Verification items for the finished model (mm, model axes). Round coordinates to 2 decimals unless told otherwise and drop trailing zeros. Loops run counter-clockwise (first coordinate to the right, second up) from the corner with the lowest first, then second, coordinate; pieces in that order, holes last. Notation, with made-up numbers: (-16, 40) - (20, 40) arc R6 cw to (20, 51) - close; hole circle Ø9 at (16.25, -15). An arc over 180 degrees is marked (long way). Use a Markdown table: item, result. Add a question column.
Autodesk Inventor part; units mm, degrees
ref_plane "YZ Plane" through (0, 0, 0) normal (1, 0, 0) x (0, 1, 0)
ref_plane "XZ Plane" through (0, 0, 0) normal (0, 1, 0) x (-1, 0, 0)
ref_plane "XY Plane" through (0, 0, 0) normal (0, 0, 1) x (1, 0, 0)
sketch "Boceto1" plane through (0, 0, 0) normal (0, 1, 0) x (-1, 0, 0)
  line L0 (-23.8, -33.6) -> (23.8, -33.6)
  line L1 (23.8, -33.6) -> (23.8, 33.6)
  line L2 (23.8, 33.6) -> (-23.8, 33.6)
  line L3 (-23.8, 33.6) -> (-23.8, -33.6)
  line L4 (-12.4, -30.6) -> (12.9, -30.6)
  line L5 (12.4, 30.6) -> (-12.9, 30.6)
  line L6 (-23.8, 33.6) -> (-23.8, 29.4)
  circle A0 centre (-18.35, 27.65) radius 1.75
  line L7 (-16.6, 29.4) -> (-20.1, 25.9) construction
  line L8 (-20.1, 29.4) -> (-16.6, 25.9) construction
  line L9 (-12.9, 22.2) -> (-20.8, 22.2)
  line L10 (-23.8, 22.2) -> (-23.8, 33.1)
  line L11 (-12.9, 30.6) -> (-12.9, 22.2)
  line L12 (0, 33.6) -> (0, -33.6)
  line L13 (-23.8, 0) -> (23.8, 0)
  circle A1 centre (-17.85, -28.15) radius 1.75
  line L14 (-19.6, -26.4) -> (-16.1, -29.9) construction
  line L15 (-19.6, -29.9) -> (-16.1, -26.4) construction
  line L16 (-12.4, -22.7) -> (-12.4, -30.6)
  line L17 (-20.8, -22.7) -> (-12.4, -22.7)
  circle A2 centre (18.35, -27.65) radius 1.75
  line L18 (16.6, -29.4) -> (20.1, -25.9) construction
  line L19 (12.9, -22.2) -> (20.8, -22.2)
  line L20 (12.9, -30.6) -> (12.9, -22.2)
  circle A3 centre (17.85, 28.15) radius 1.75
  line L21 (19.6, 26.4) -> (16.1, 29.9) construction
  line L22 (19.6, 29.9) -> (16.1, 26.4) construction
  line L23 (12.4, 22.7) -> (12.4, 30.6)
  line L24 (20.8, 22.7) -> (12.4, 22.7)
  line L25 (20.8, -22.2) -> (20.8, 22.7)
  line L26 (-20.8, 22.2) -> (-20.8, -22.7)
  point P0 (0, 0)
  dimension "d0" = 47.6
  dimension "d1" = 67.2
  dimension "d3" = 4.2
  dimension "d5" = 3.5
  dimension "d9" = 3.5
  dimension "d11" = 3.5
extrude "Extrusión1" add sketch "Boceto1" along normal blind 2 contours L3 L13 L26 L17 L16 L4 L12 L0 | L12 L4 L20 L19 L25 L13 L1 L0 | L3 L2 L12 L5 L11 L9 L26 L13 | L13 L25 L24 L23 L5 L12 L2 L1
fillet "Empalme1" radius 8.4 4 edges at (-12.4, 1, 22.7) (12.9, 1, 22.2) (12.4, 1, -22.7) (-12.9, 1, -22.2)
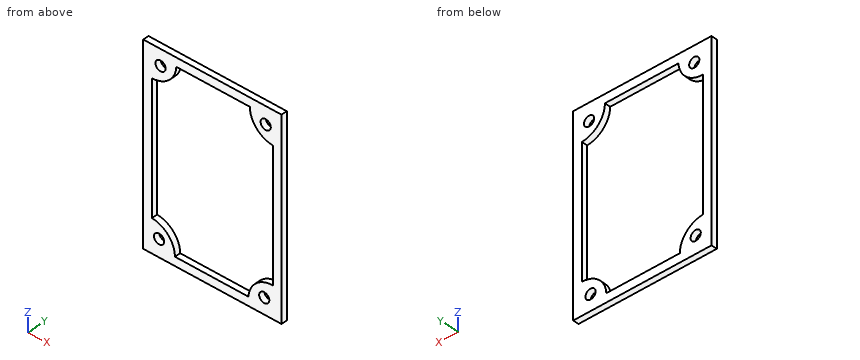
Q1. Section check D-D on x = -18.35. Record the cut outline in (y, z), plus the area to 3 significant figures.
Q2. Section check A-A on y = 0.8. State how many separate pieces and enclosed holes the cut face has, plus the area to 3 significant figures.
Q3. Section check C-C on z = -3.5. Record the cut outline in (x, y), plus the area to 3 significant figures.
Q4. Thickness scan on line 1 along X through (y, z) = (1.1, 5); line 2 along Z through (x, y) = (-17.85, 0.6); line 3 along Z through (x, y) = (18, 1.85). Record the ranges inside material, lowest first.
Q5. Section check B-B on x = -10. Record the cut outline in (y, z).
Determined:
| question | item | result |
|---|---|---|
| 1 | outline | (0, -33.6) - (2, -33.6) - (2, -29.4) - (0, -29.4) - close; (0, -25.9) - (2, -25.9) - (2, -22.72) - (0, -22.72) - close; (0, 23.06) - (2, 23.06) - (2, 26.47) - (0, 26.47) - close; (0, 29.83) - (2, 29.83) - (2, 33.6) - (0, 33.6) - close |
| 1 | area | 29.1 mm² |
| 2 | separate pieces | 1 |
| 2 | enclosed holes | 5 |
| 2 | area | 820 mm² |
| 3 | outline | (-23.8, 0) - (-20.8, 0) - (-20.8, 2) - (-23.8, 2) - close; (20.8, 0) - (23.8, 0) - (23.8, 2) - (20.8, 2) - close |
| 3 | area | 12.0 mm² |
| 4 | line 1 | x = -23.8 to -20.8, 20.8 to 23.8 |
| 4 | line 2 | z = -33.6 to -29.33, -25.97 to -22.93, 23.23 to 26.4, 29.9 to 33.6 |
| 4 | line 3 | z = -33.6 to -29.89, -26.41 to -23.18, 22.86 to 25.94, 29.36 to 33.6 |
| 5 | outline | (0, -33.6) - (2, -33.6) - (2, -30.6) - (0, -30.6) - close; (0, 30.6) - (2, 30.6) - (2, 33.6) - (0, 33.6) - close |
